```python
from build123d import *

# Parameters (mm, degrees)
SKETCH_1_W          = 80
SKETCH_1_H          = 40
EXTRUDE_1_DEPTH     = 500
SKETCH_2_W          = 400
SKETCH_2_H          = 40
EXTRUDE_2_DEPTH     = 40
SKETCH_3_W          = 400
SKETCH_3_H          = 40
EXTRUDE_3_DEPTH     = 40
CUT_EXTRUDE_1_DEPTH = 121
SKETCH_5_W          = 40
SKETCH_5_H          = 150
EXTRUDE_4_DEPTH     = 40
SKETCH_6_W          = 40
SKETCH_6_H          = 40
EXTRUDE_5_DEPTH     = 100
SKETCH_7_W          = 40
SKETCH_7_H          = 150
EXTRUDE_6_DEPTH     = 40
SKETCH_8_W          = 40
SKETCH_8_H          = 40
EXTRUDE_7_DEPTH     = 100
SKETCH_9_W          = 40
SKETCH_9_H          = 150
EXTRUDE_8_DEPTH     = 40
SKETCH_10_W         = 40
SKETCH_10_H         = 40
EXTRUDE_9_DEPTH     = 100
CUT_EXTRUDE_2_DEPTH = 121
SKETCH_13_W         = 301.005050634
SKETCH_13_H         = 40
EXTRUDE_10_DEPTH    = 40
SKETCH_14_W         = 40
SKETCH_14_H         = 40
EXTRUDE_11_DEPTH    = 500
SKETCH_15_W         = 80
SKETCH_15_H         = 40
EXTRUDE_12_DEPTH    = 146.066017
EXTRUDE_13_REACH    = 411.497
SKETCH_17_W         = 40
SKETCH_17_H         = 40
CUT_EXTRUDE_3_DEPTH = 500
SKETCH_19_W         = 80
SKETCH_19_H         = 40
EXTRUDE_14_DEPTH    = 500
SKETCH_20_W         = 80
SKETCH_20_H         = 40
EXTRUDE_15_DEPTH    = 300
SKETCH_21_W         = 40
SKETCH_21_H         = 40
EXTRUDE_16_DEPTH    = 300
SKETCH_22_W         = 80
SKETCH_22_H         = 40
EXTRUDE_17_DEPTH    = 300
SKETCH_23_W         = 40
SKETCH_23_H         = 40
EXTRUDE_18_DEPTH    = 300
EXTRUDE_19_DEPTH    = 40
EXTRUDE_20_DEPTH    = 40
EXTRUDE_21_DEPTH    = 80
EXTRUDE_22_DEPTH    = 80


with BuildPart() as part:
    # 草图1 → 凸台-拉伸1 (new body)
    with BuildSketch(Plane(origin=(0, 0, 0), x_dir=(1, 0, 0), z_dir=(0, 1, 0))):
        with Locations((40, -20)):
            Rectangle(SKETCH_1_W, SKETCH_1_H)
    extrude(amount=EXTRUDE_1_DEPTH)

    # 草图2 → 凸台-拉伸2 (add)
    with BuildSketch(Plane.XY.offset(40)):
        with Locations((40, 480)):
            Rectangle(SKETCH_2_W, SKETCH_2_H)
    extrude(amount=EXTRUDE_2_DEPTH)

    # 草图3 → 凸台-拉伸3 (add)
    with BuildSketch(Plane(origin=(0, 0, 0), x_dir=(-1, 0, 0), z_dir=(0, 0, -1))):
        with Locations((-40, 480)):
            Rectangle(SKETCH_3_W, SKETCH_3_H)
    extrude(amount=EXTRUDE_3_DEPTH)

    # 草图4 → 切除-拉伸1 (cut, through all)
    with BuildSketch(Plane.XY.offset(80)):
        Polygon((-160, 500), (-120, 460), (-160, 460), align=None)
        Polygon((240, 500), (200, 460), (240, 460), align=None)
    extrude(amount=-CUT_EXTRUDE_1_DEPTH, mode=Mode.SUBTRACT)

    # 草图5 → 凸台-拉伸4 (add)
    with BuildSketch(Plane(origin=(-130, 130, 0), x_dir=(0, 0, -1), z_dir=(0.707106781, -0.707106781, 0))):
        with Locations((-60, 448.259018078)):
            Rectangle(SKETCH_5_W, SKETCH_5_H)
    extrude(amount=EXTRUDE_4_DEPTH)

    # 草图6 → 凸台-拉伸5 (add)
    with BuildSketch(Plane(origin=(370, 370, 0), x_dir=(0, 0, -1), z_dir=(0.707106781, 0.707106781, 0))):
        with Locations((-60, 163.847763108)):
            Rectangle(SKETCH_6_W, SKETCH_6_H)
    extrude(amount=EXTRUDE_5_DEPTH)

    # 草图7 → 凸台-拉伸6 (add)
    with BuildSketch(Plane(origin=(-130, 130, 0), x_dir=(0, 0, -1), z_dir=(0.707106781, -0.707106781, 0))):
        with Locations((20, 448.259018078)):
            Rectangle(SKETCH_7_W, SKETCH_7_H)
    extrude(amount=EXTRUDE_6_DEPTH)

    # 草图8 → 凸台-拉伸7 (add)
    with BuildSketch(Plane(origin=(370, 370, 0), x_dir=(0, 0, -1), z_dir=(0.707106781, 0.707106781, 0))):
        with Locations((20, 163.847763108)):
            Rectangle(SKETCH_8_W, SKETCH_8_H)
    extrude(amount=EXTRUDE_7_DEPTH)

    # 草图9 → 凸台-拉伸8 (add)
    with BuildSketch(Plane(origin=(170, 170, 0), x_dir=(0, 0, 1), z_dir=(-0.707106781, -0.707106781, 0))):
        with Locations((-20, 391.690475583)):
            Rectangle(SKETCH_9_W, SKETCH_9_H)
        with Locations((60, 391.690475583)):
            Rectangle(SKETCH_9_W, SKETCH_9_H)
    extrude(amount=EXTRUDE_8_DEPTH)

    # 草图10 → 凸台-拉伸9 (add)
    with BuildSketch(Plane(origin=(-330, 330, 0), x_dir=(0, 0, 1), z_dir=(-0.707106781, 0.707106781, 0))):
        with Locations((-20, 220.416305603)):
            Rectangle(SKETCH_10_W, SKETCH_10_H)
        with Locations((60, 220.416305603)):
            Rectangle(SKETCH_10_W, SKETCH_10_H)
    extrude(amount=EXTRUDE_9_DEPTH)

    # 草图12 → 切除-拉伸2 (cut, through all)
    with BuildSketch(Plane.XY.offset(80)):
        Polygon((-82.218254069, 365.649711575), (-53.933982822, 393.933982822), (-110.502525317, 393.933982822), align=None)
        Polygon((133.933982822, 393.933982822), (162.218254069, 365.649711575), (190.502525317, 393.933982822), align=None)
    extrude(amount=-CUT_EXTRUDE_2_DEPTH, mode=Mode.SUBTRACT)

    # 草图13 → 凸台-拉伸10 (add)
    with BuildSketch(Plane.XZ.offset(-393.933982822)):
        with Locations((40, 60)):
            Rectangle(SKETCH_13_W, SKETCH_13_H)
        with Locations((40, -20)):
            Rectangle(SKETCH_13_W, SKETCH_13_H)
    extrude(amount=EXTRUDE_10_DEPTH)

    # 草图14 → 凸台-拉伸11 (add)
    with BuildSketch(Plane(origin=(0, 353.933982822, 0), x_dir=(-1, 0, 0), z_dir=(0, -1, 0))):
        with Locations((90.502525317, -60)):
            Rectangle(SKETCH_14_W, SKETCH_14_H)
        with Locations((90.502525317, 20)):
            Rectangle(SKETCH_14_W, SKETCH_14_H)
        with Locations((-170.502525317, -60)):
            Rectangle(SKETCH_14_W, SKETCH_14_H)
        with Locations((-170.502525317, 20)):
            Rectangle(SKETCH_14_W, SKETCH_14_H)
    extrude(amount=EXTRUDE_11_DEPTH)

    # 草图15 → 凸台-拉伸12 (add)
    with BuildSketch(Plane.XZ):
        with Locations((40, 20)):
            Rectangle(SKETCH_15_W, SKETCH_15_H)
    extrude(amount=EXTRUDE_12_DEPTH)

    # 草图17 → 凸台-拉伸13 (add, up to next)
    with BuildSketch(Plane(origin=(-70.502525317, 0, 0), x_dir=(0, 0, -1), z_dir=(1, 0, 0)), mode=Mode.PRIVATE) as extrude_13_sk1:
        with Locations((-60, -126.066017178)):
            Rectangle(SKETCH_17_W, SKETCH_17_H)
    extrude_13_tool1 = extrude(extrude_13_sk1.sketch, amount=EXTRUDE_13_REACH, mode=Mode.PRIVATE) - part.part
    add(extrude_13_tool1.solids().sort_by_distance((-70.502525, -126.066017, 60))[0])
    # 草图17 → 凸台-拉伸13 (add, up to next)
    with BuildSketch(Plane(origin=(-70.502525317, 0, 0), x_dir=(0, 0, -1), z_dir=(1, 0, 0)), mode=Mode.PRIVATE) as extrude_13_sk2:
        with Locations((20, -126.066017178)):
            Rectangle(SKETCH_17_W, SKETCH_17_H)
    extrude_13_tool2 = extrude(extrude_13_sk2.sketch, amount=EXTRUDE_13_REACH, mode=Mode.PRIVATE) - part.part
    add(extrude_13_tool2.solids().sort_by_distance((-70.502525, -126.066017, -20))[0])

    # 草图18 → 切除-拉伸3 (cut)
    with BuildSketch(Plane.XZ.offset(146.066017178)):
        Polygon((-110.502525317, 80), (-110.502525317, 40), (0, 40), (0, 0), (-110.502525317, 0), (-110.502525317, -40), (190.502525317, -40), (190.502525317, 0), (80, 0), (80, 40), (190.502525317, 40), (190.502525317, 80), align=None)
    extrude(amount=-CUT_EXTRUDE_3_DEPTH, mode=Mode.SUBTRACT)

    # 草图19 → 凸台-拉伸14 (add)
    with BuildSketch(Plane.XZ.offset(-353.933982822)):
        with Locations((40, 20)):
            Rectangle(SKETCH_19_W, SKETCH_19_H)
    extrude(amount=EXTRUDE_14_DEPTH)

    # 草图20 → 凸台-拉伸15 (add)
    with BuildSketch(Plane.XY.offset(40)):
        with Locations((40, -126.066017178)):
            Rectangle(SKETCH_20_W, SKETCH_20_H)
    extrude(amount=EXTRUDE_15_DEPTH)

    # 草图21 → 凸台-拉伸16 (add)
    with BuildSketch(Plane(origin=(80, 0, 0), x_dir=(0, 0, -1), z_dir=(1, 0, 0))):
        with Locations((-20, -126.066017178)):
            Rectangle(SKETCH_21_W, SKETCH_21_H)
    extrude(amount=EXTRUDE_16_DEPTH)

    # 草图22 → 凸台-拉伸17 (add)
    with BuildSketch(Plane(origin=(0, 0, 0), x_dir=(-1, 0, 0), z_dir=(0, 0, -1))):
        with Locations((-40, -126.066017178)):
            Rectangle(SKETCH_22_W, SKETCH_22_H)
    extrude(amount=EXTRUDE_17_DEPTH)

    # 草图23 → 凸台-拉伸18 (add)
    with BuildSketch(Plane.ZY):
        with Locations((20, -126.066017178)):
            Rectangle(SKETCH_23_W, SKETCH_23_H)
    extrude(amount=EXTRUDE_18_DEPTH)

    # 草图24 → 凸台-拉伸19 (add)
    with BuildSketch(Plane.XY.offset(40)):
        Polygon((-243.431457505, -106.066017178), (0, 137.365440327), (0, 193.933982822), (-300, -106.066017178), align=None)
    extrude(amount=-EXTRUDE_19_DEPTH)

    # 草图25 → 凸台-拉伸20 (add)
    with BuildSketch(Plane.XY.offset(40)):
        Polygon((380, -106.066017178), (80, 193.933982822), (80, 137.365440327), (323.431457505, -106.066017178), align=None)
    extrude(amount=-EXTRUDE_20_DEPTH)

    # 草图26 → 凸台-拉伸21 (add)
    with BuildSketch(Plane.ZY):
        Polygon((-300, -106.066017178), (0, 193.933982822), (0, 137.365440327), (-243.431457505, -106.066017178), align=None)
    extrude(amount=-EXTRUDE_21_DEPTH)

    # 草图27 → 凸台-拉伸22 (add)
    with BuildSketch(Plane.ZY):
        Polygon((340, -106.066017178), (40, 193.933982822), (40, 137.365440327), (283.431457505, -106.066017178), align=None)
    extrude(amount=-EXTRUDE_22_DEPTH)


solid = part.part
```
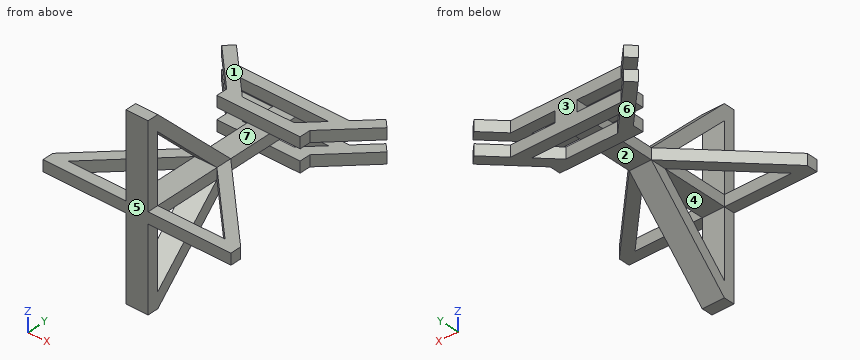
Can you work these out from the model? Positions are in its coordinate system, mm. Face numbers are marked on the shaded views. A direction names the side the tool comes from. Round coordinates to 2 decimals unless told otherwise and drop trailing zeros. Loops run counter-clockwise (first coordinate to the right, second up) from the corner with the lowest first, then second, coordinate; pieces in that order, holes last.
Item 1: If we mould it in two halves opening along Y, with no side actions, what happens to the marked faces 5, 6 and 7? For each: +Y half, -Y half, draft (parallel to the pull), parting line (faces both ways), or undercut.
Item 2: Suppose I cut it at A-A, the plane x = 52. Write out the boundary of the cut face in (y, z).
Item 3: Please list where these lines run through material, in increasing order: L1, parallel to Z at x = 110.5, y = 377.5; L2, parallel to Y at x = 154, z = -18.5; L3, parallel to X at y = 138, z = 50.
Item 4: Suppose I cut it at C-C, the plane y = -79.5. Write out the boundary of the cut face in (x, z).
Item 5: Suppose I cut it at D-D, the plane z = -84. Write out the boundary of the cut face in (x, y).
Item 6: Which directions (+Z, -Z, +X, -X, +Y, -Y) give clear straight access to the entire face, cutting with the end or side of a thin tool? Please do the marked faces 1, 2, 3 and 4.
Item 7: Suppose I cut it at B-B, the plane x = 217. Write out the boundary of the cut face in (y, z), then the cut area to 3 significant figures.
Item 8: Will these pins go through, and if not, where does the flat tip stop? pin 1 Ø3 at (x, y) = (-70, 399) entering from -Z; pin 2 Ø20 at (x, z) = (-20.5, 67.5) entering from -Y; pin 3 Ø12 at (y, z) = (377, -22.5) entering from -X.
Reported:
1. face 5: -Y half
1. face 6: draft
1. face 7: undercut
2. outline: (-146.07, -300) - (-106.07, -300) - (193.93, 0) - (353.93, 0) - (353.93, -40) - (393.93, -40) - (393.93, 0) - (460, 0) - (460, -40) - (500, -40) - (500, 80) - (460, 80) - (460, 40) - (393.93, 40) - (393.93, 80) - (353.93, 80) - (353.93, 40) - (193.93, 40) - (-106.07, 340) - (-146.07, 340) - close; hole (-106.07, -243.43) - (137.37, 0) - (-106.07, 0) - close; hole (-106.07, 40) - (137.37, 40) - (-106.07, 283.43) - close
3. L1: z = -40 to 0, 40 to 80
3. L2: y = 353.93 to 414, 460 to 500
3. L3: x = 0 to 80
4. outline: (-273.43, 0) - (-216.87, 0) - (-216.87, 40) - (-273.43, 40) - close; (0, -273.43) - (80, -273.43) - (80, -216.87) - (0, -216.87) - close; (0, 0) - (80, 0) - (80, 40) - (0, 40) - close; (0, 256.87) - (80, 256.87) - (80, 313.43) - (0, 313.43) - close; (296.87, 0) - (353.43, 0) - (353.43, 40) - (296.87, 40) - close
5. outline: (0, -146.07) - (80, -146.07) - (80, -106.07) - (0, -106.07) - close; (0, 53.37) - (80, 53.37) - (80, 109.93) - (0, 109.93) - close
6. face 1: +Z, +X, -X, +Y
6. face 2: -Z, +X, -X
6. face 3: +Z, -Z, +Y
6. face 4: +X, -X
7. outline: (-146.07, 0) - (-106.07, 0) - (-106.07, 40) - (-146.07, 40) - close; (0.37, 0) - (56.93, 0) - (56.93, 40) - (0.37, 40) - close; (420.43, -40) - (500, -40) - (500, 0) - (420.43, 0) - close; (420.43, 40) - (500, 40) - (500, 80) - (420.43, 80) - close
7. area: 10,200 mm2
8. pin 1: stops at z = -40
8. pin 2: stops at y = 353.93
8. pin 3: stops at x = -110.5
